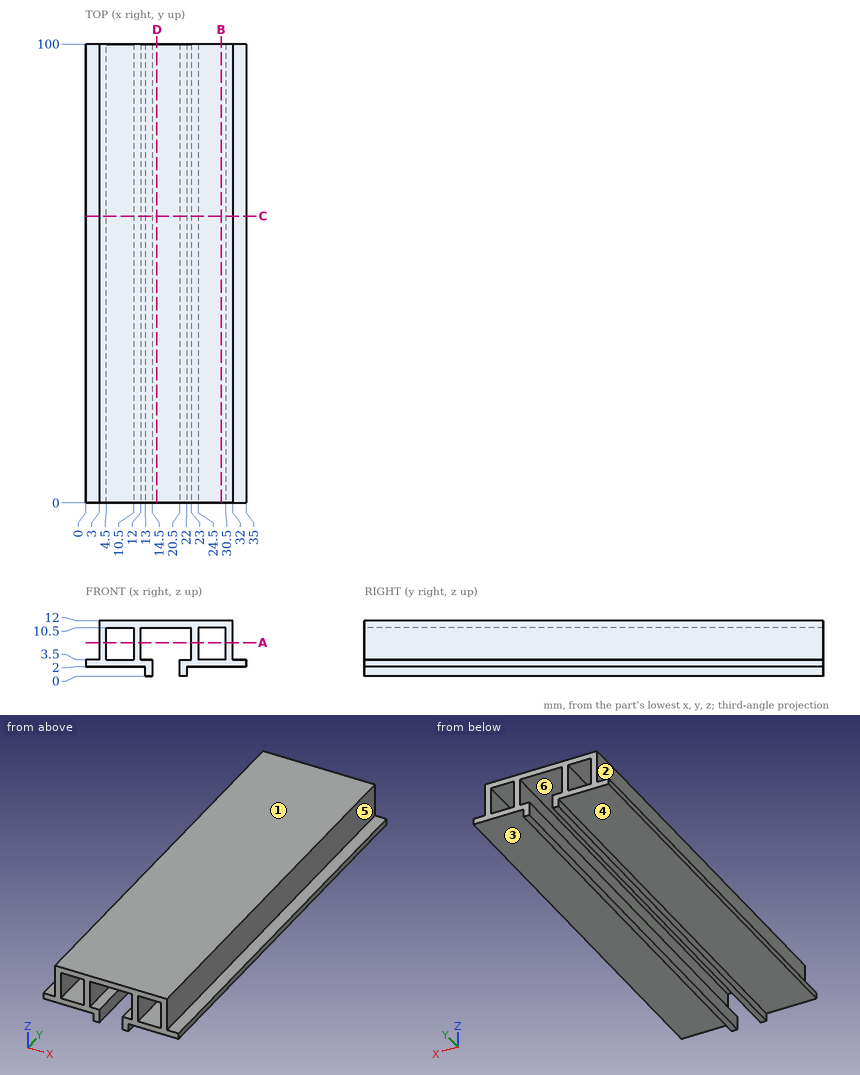
Geometry check sheet. Reference: drawing and pictorial views, mm from the part's lowest x, y, z. A direction names the side the tool comes from. Round coordinates to 2 decimals unless told otherwise and drop trailing zeros. Loops run counter-clockwise (first coordinate to the right, second up) from the corner with the lowest first, then second, coordinate; pieces in that order, holes last. Notation, with made-up numbers: (16, 86.25) -> (70, 86.25) arc R34 ccw to (70, 123.25) -> close; hole circle Ø11 at (84, 77). An arc over 180 degrees is marked (long way). Answer as a JSON object with one key per item and string values. Group by question number.
Item 1: Cross-section at D-D, the plane x = 15.5. Record the cut outline in (y, z).
Item 2: Cross-section at A-A, the plane z = 7.25. Record the cut outline in (x, y), plus the area to 3 significant figures.
Item 3: Cross-section at B-B, the plane x = 29.5. Record the cut outline in (y, z), plus the area to 3 significant figures.
Item 4: Cross-section at C-C, the plane y = 62.5. Record the cut outline in (x, z), plus the area to 3 significant figures.
Item 5: Release check for a two-part mould opening along Z. For the marked faces 4, 5 and 6 record: pulls with the +Z half, pulls with the -Z half, needs draft (parallel to the pull), parting line crosses it, or undercut.
Item 6: Set-up check for the marked faces 1, 2 and 3: record each of +Z, -Z, +X, -X, +Y, -Y from which the full face is reachable in a straight line by a thin tool's end or side.
Item 7: Thickness scan on line 1 along X through (y, z) = (82.5, 9.5); line 2 along X through (y, z) = (51.5, 1.5); line 3 along X through (y, z) = (39, 3.25). Record the ranges inside material, lowest first.
Item 8: Depth check by flat-ended pin: pin 1 Ø5 at (x, y) = (29, 60) entering from -Z; pin 2 Ø1 at (y, z) = (33, 1) entering from -X; pin 3 Ø1 at (y, z) = (36, 1) entering from +X. Enter the tip coordinate at first touch or a pass-through.
Determined:
{
 "1": {"outline": "(0, 10.5) -> (100, 10.5) -> (100, 12) -> (0, 12) -> close"},
 "2": {"outline": "(3, 0) -> (4.5, 0) -> (4.5, 100) -> (3, 100) -> close; (10.5, 0) -> (12, 0) -> (12, 100) -> (10.5, 100) -> close; (23, 0) -> (24.5, 0) -> (24.5, 100) -> (23, 100) -> close; (30.5, 0) -> (32, 0) -> (32, 100) -> (30.5, 100) -> close", "area": "600 mm²"},
 "3": {"outline": "(0, 2) -> (100, 2) -> (100, 3.5) -> (0, 3.5) -> close; (0, 10.5) -> (100, 10.5) -> (100, 12) -> (0, 12) -> close", "area": "300 mm²"},
 "4": {"outline": "(0, 2) -> (13, 2) -> (13, 0) -> (14.5, 0) -> (14.5, 3.5) -> (12, 3.5) -> (12, 10.5) -> (23, 10.5) -> (23, 3.5) -> (20.5, 3.5) -> (20.5, 0) -> (22, 0) -> (22, 2) -> (35, 2) -> (35, 3.5) -> (32, 3.5) -> (32, 12) -> (3, 12) -> (3, 3.5) -> (0, 3.5) -> close; hole (4.5, 3.5) -> (10.5, 3.5) -> (10.5, 10.5) -> (4.5, 10.5) -> close; hole (24.5, 3.5) -> (30.5, 3.5) -> (30.5, 10.5) -> (24.5, 10.5) -> close", "area": "135 mm²"},
 "5": {"face 4": "pulls with the -Z half", "face 5": "needs draft", "face 6": "undercut"},
 "6": {"face 1": "+Z, +X, -X, +Y, -Y", "face 2": "+Z, -X, +Y, -Y", "face 3": "-Z, +X, +Y, -Y"},
 "7": {"line 1": "x = 3 to 4.5, 10.5 to 12, 23 to 24.5, 30.5 to 32", "line 2": "x = 13 to 14.5, 20.5 to 22", "line 3": "x = 0 to 14.5, 20.5 to 35"},
 "8": {"pin 1": "stops at z = 2", "pin 2": "stops at x = 13", "pin 3": "stops at x = 22"}
}
